```python
from build123d import *

# Parameters (mm, degrees)
SKETCH2_W           = 89
SKETCH2_H           = 89
BOSS_EXTRUDE1_DEPTH = 40
SKETCH5_W           = 80
SKETCH5_H           = 80
CUT_EXTRUDE3_DEPTH  = 10
SKETCH4_W           = 80
SKETCH4_H           = 80
CUT_EXTRUDE5_DEPTH  = 10
CUT_EXTRUDE6_DEPTH  = 3.5
CIRPATTERN1_COUNT   = 4
FILLET1_R           = 0.5


with BuildPart() as part:
    # Sketch2 → Boss-Extrude1 (new body)
    with BuildSketch(Plane(origin=(0, 0, 0), x_dir=(1, 0, 0), z_dir=(0, 1, 0))):
        Rectangle(SKETCH2_W, SKETCH2_H)
    extrude(amount=BOSS_EXTRUDE1_DEPTH)

    # Sketch5 → Cut-Extrude3 (cut)
    with BuildSketch(Plane.XZ):
        Rectangle(SKETCH5_W, SKETCH5_H)
    extrude(amount=-CUT_EXTRUDE3_DEPTH, mode=Mode.SUBTRACT)

    # Sketch4 → Cut-Extrude5 (cut)
    with BuildSketch(Plane(origin=(0, 40, 0), x_dir=(1, 0, 0), z_dir=(0, 1, 0))):
        Rectangle(SKETCH4_W, SKETCH4_H)
    extrude(amount=-CUT_EXTRUDE5_DEPTH, mode=Mode.SUBTRACT)

    # Sketch6 → Cut-Extrude6 (cut)
    with BuildSketch(Plane(origin=(44.5, 0, 0), x_dir=(0, 0, -1), z_dir=(1, 0, 0))):
        with BuildLine():
            ThreePointArc((3, 20), (2.121320344, 22.121320344), (0, 23))
            Line((0, 23), (0, 17))
            ThreePointArc((0, 17), (2.121320344, 17.878679656), (3, 20))
        make_face()
        with BuildLine():
            Line((0, 17), (0, 23))
            ThreePointArc((0, 23), (-3, 20), (0, 17))
        make_face()
    cut_extrude6 = extrude(amount=-CUT_EXTRUDE6_DEPTH, mode=Mode.SUBTRACT)

    # CirPattern1: Cut-Extrude6 ×4 about axis
    cirpattern1_axis = Axis((0, 10, 0), (0, -1, 0))
    for i in range(1, CIRPATTERN1_COUNT):
        add(cut_extrude6.rotate(cirpattern1_axis, i * 360 / CIRPATTERN1_COUNT), mode=Mode.SUBTRACT)

    # Fillet1
    fillet1_edges = [part.edges().sort_by_distance(p)[0] for p in [
        (-44.5, 40, 0),
        (0, 40, 44.5),
        (40, 5, 40),
        (40, 5, -40),
        (-40, 5, -40),
        (-40, 5, 40),
        (40, 0, 0),
        (0, 0, 40),
        (-40, 0, 0),
        (0, 0, -40),
        (40, 35, -40),
        (40, 35, 40),
        (-40, 35, 40),
        (-40, 35, -40),
        (40, 40, 0),
        (0, 40, -40),
        (-40, 40, 0),
        (0, 40, 40),
        (44.5, 40, 0),
        (0, 0, 44.5),
        (-44.5, 0, 0),
        (0, 0, -44.5),
        (44.5, 0, 0),
        (44.5, 20, 44.5),
        (-44.5, 20, 44.5),
        (-44.5, 20, -44.5),
        (44.5, 20, -44.5),
        (0, 40, -44.5),
    ]]
    fillet(fillet1_edges, radius=FILLET1_R)


solid = part.part
```
Work out the finished part from the listing and answer in its coordinate system (mm). A direction names the side the tool comes from. Give positions to 0.01 mm unless a question says otherwise; leave off trailing zeros. Order: outer loops, then holes, each group sorted by start corner. A loop starts at its lowest first (then second) coordinate and runs counter-clockwise, first axis right, second up.
1. For faces 4 (the flat face through (-1, 30, -1)), 5 (the flat face through (-41, 20, 0)), 6 (the flat face through (-1, 5, -40)), determine the directions among +Z, -Z, +X, -X, +Y, -Y from which every point of the face is accessible in a straight line to the end or side of a thin tool.
Result sheet:
face 4: +Y
face 5: -X
face 6: -Y
2. Section A-A, the plane x = -14 is taken. Determine the outline of the cut face in (y, z), and give its area (3 significant figures).
Result sheet:
outline: (0, -44) arc R0.5 ccw to (0.5, -44.5) - (39.5, -44.5) arc R0.5 ccw to (40, -44) - (40, -40.5) arc R0.5 ccw to (39.5, -40) - (30, -40) - (30, 40) - (39.5, 40) arc R0.5 ccw to (40, 40.5) - (40, 44) arc R0.5 ccw to (39.5, 44.5) - (0.5, 44.5) arc R0.5 ccw to (0, 44) - (0, 40.5) arc R0.5 ccw to (0.5, 40) - (10, 40) - (10, -40) - (0.5, -40) arc R0.5 ccw to (0, -40.5) - close
area: 1,960 mm2
3. Each of these flat-tipped pins is pushed along its axis until it touches: P1, Ø5, axis at y = 18.5, z = 0.5, coming from the +X side; P2, Ø3, axis at x = -31.5, z = 25, coming from the -Y side; P3, Ø8, axis at x = 4.5, z = 6, coming from the +Y side; P4, Ø1.8, axis at x = 1.5, y = 19.5, coming from the -Z side. Where does it stop, or does it pass through?
Result sheet:
P1: stops at x = 44.5
P2: stops at y = 10
P3: stops at y = 30
P4: stops at z = -41
4. Straight lines are drawn through the part: L1, parallel to X at y = 4, z = 26; L2, parallel to Y at x = 18.5, z = -2.5. For each, find the intervals that lie inside material, in ascending order.
Result sheet:
L1: x = -44.5 to -40, 40 to 44.5
L2: y = 10 to 30
5. The mould has two halves that part along X. Classify faces 1 (the flat face through (-3, 0, 42)), 2 (the flat face through (-1, 35, 40)), 3 (the flat face through (44.5, 24, 1)): released by +X, released by -X, zero draft, split by the parting line, or undercut.
Result sheet:
face 1: zero draft
face 2: undercut
face 3: released by +X
6. Section B-B, the plane z = 17.5 is taken. Determine the outline of the cut face in (x, y), and give its area (3 significant figures).
Result sheet:
outline: (-44.5, 0.5) arc R0.5 ccw to (-44, 0) - (-40.5, 0) arc R0.5 ccw to (-40, 0.5) - (-40, 10) - (40, 10) - (40, 0.5) arc R0.5 ccw to (40.5, 0) - (44, 0) arc R0.5 ccw to (44.5, 0.5) - (44.5, 39.5) arc R0.5 ccw to (44, 40) - (40.5, 40) arc R0.5 ccw to (40, 39.5) - (40, 30) - (-40, 30) - (-40, 39.5) arc R0.5 ccw to (-40.5, 40) - (-44, 40) arc R0.5 ccw to (-44.5, 39.5) - close
area: 1,960 mm2
